from build123d import *

# Parameters (mm, degrees)
SKETCH1_R           = 0.75
SKETCH1_R_2         = 0.5
BOSS_EXTRUDE1_DEPTH = 2


with BuildPart() as part:
    # Sketch1 → Boss-Extrude1 (new body)
    with BuildSketch(Plane.XY):
        with BuildLine():
            Line((0, 16), (0, 14))
            Line((0, 14), (4, 14))
            Line((4, 14), (4, 12))
            Line((4, 12), (0, 12))
            Line((0, 12), (0, 6))
            Line((0, 6), (4, 6))
            Line((4, 6), (4, 4))
            Line((4, 4), (0, 4))
            Line((0, 4), (0, 2))
            ThreePointArc((0, 2), (0.585786438, 0.585786438), (2, 0))
            Line((2, 0), (14.2, 0))
            ThreePointArc((14.2, 0), (15.614213562, 0.585786438), (16.2, 2))
            Line((16.2, 2), (16.2, 4))
            Line((16.2, 4), (12.2, 4))
            Line((12.2, 4), (12.2, 6))
            Line((12.2, 6), (16.2, 6))
            Line((16.2, 6), (16.2, 12))
            Line((16.2, 12), (12.2, 12))
            Line((12.2, 12), (12.2, 14))
            Line((12.2, 14), (16.2, 14))
            Line((16.2, 14), (16.2, 16))
            ThreePointArc((16.2, 16), (14.735533906, 19.535533906), (11.2, 21))
            Line((11.2, 21), (5, 21))
            ThreePointArc((5, 21), (1.464466094, 19.535533906), (0, 16))
        make_face()
        with Locations((10.2, 8.5)):
            Circle(SKETCH1_R, mode=Mode.SUBTRACT)
        with Locations((6, 8.5)):
            Circle(SKETCH1_R, mode=Mode.SUBTRACT)
        with Locations((3, 18)):
            Circle(SKETCH1_R_2, mode=Mode.SUBTRACT)
        with Locations((13.2, 18)):
            Circle(SKETCH1_R_2, mode=Mode.SUBTRACT)
        with Locations((13.45, 2)):
            Circle(SKETCH1_R, mode=Mode.SUBTRACT)
        with Locations((2.75, 2)):
            Circle(SKETCH1_R, mode=Mode.SUBTRACT)
    extrude(amount=BOSS_EXTRUDE1_DEPTH)


solid = part.part
Can you work these out from the model? Positions are in its coordinate system, mm. A direction names the side the tool comes from. Coordinates: 2 decimals unless noted, no trailing zeros. Write each loop counter-clockwise with the first axis right and the second up, starting at its lowest first coordinate (ties: lowest second). Pieces come first, ordered by that corner, then holes. Notation, with made-up numbers: (14.25, 83.5) -> (49.25, 83.5) arc R20 cw to (49.25, 111.5) -> close; hole circle Ø4 at (79.5, -8.75). An arc over 180 degrees is marked (long way). Write item = value, one per line.
(1) On a 3-axis mill with a long thin cutter (end or side, diameter ignored), from which of +Z, -Z, +X, -X, +Y, -Y can I reach the whole of each face in a straight line? I mean faces 1 (the face through (8, 11, 2)), 2 (the face through (12.2, 13, 1)), 3 (the face through (2, 6, 1)). Say none if no direction works.
Verdict:
face_1 = +Z, +X, -X, +Y, -Y
face_2 = +Z, -Z, +X
face_3 = +Z, -Z, -X
(2) For pin 1 (0.6 mm diameter, centred on y = 12.5, z = 0.5, fed in from -X); pin 2 (1 mm diameter, centred on x = 2.5, z = 1, fed in from +Y); pin 3 (1 mm diameter, centred on x = 15, z = 0.5, fed in from +Y), each with a flat end and sliding along its axis, tell me the tip position at first contact or that it passes through.
Verdict:
pin_1 = 4
pin_2 = 20.58
pin_3 = 19.76
(3) Imagine slicing it at D-D (x = 2.75). Please give me the cut outline in (y, z), and give its area (3 significant figures).
Verdict:
outline = (0, 0) -> (1.25, 0) -> (1.25, 2) -> (0, 2) -> close; (2.75, 0) -> (4, 0) -> (4, 2) -> (2.75, 2) -> close; (6, 0) -> (12, 0) -> (12, 2) -> (6, 2) -> close; (14, 0) -> (17.57, 0) -> (17.57, 2) -> (14, 2) -> close; (18.43, 0) -> (20.47, 0) -> (20.47, 2) -> (18.43, 2) -> close
area = 28.2 mm^2
(4) Imagine slicing it at C-C (x = 6). Please give me the cut outline in (y, z), and give its area (3 significant figures).
Verdict:
outline = (0, 0) -> (7.75, 0) -> (7.75, 2) -> (0, 2) -> close; (9.25, 0) -> (21, 0) -> (21, 2) -> (9.25, 2) -> close
area = 39.0 mm^2
(5) If I drill on probe 1 along Y at (x, z) = (10.2, 0.8); probe 2 along Y at (x, z) = (14.25, 0.8); probe 3 along X at (y, z) = (13.75, 0.3), over which ranges is the centre line in solid material (lowest first)?
Verdict:
probe_1 = 0 to 7.75, 9.25 to 21
probe_2 = 0 to 4, 6 to 12, 14 to 19.96
probe_3 = 4 to 12.2
(6) Imagine slicing it at B-B (y = 8.5). Please give me the cut outline in (x, z), and give its area (3 significant figures).
Verdict:
outline = (0, 0) -> (5.25, 0) -> (5.25, 2) -> (0, 2) -> close; (6.75, 0) -> (9.45, 0) -> (9.45, 2) -> (6.75, 2) -> close; (10.95, 0) -> (16.2, 0) -> (16.2, 2) -> (10.95, 2) -> close
area = 26.4 mm^2
(7) Imagine slicing it at A-A (z = 1.45). State how many separate pieces and enclosed holes the cut face has, and give its area (3 significant figures).
Verdict:
separate_pieces = 1
enclosed_holes = 6
area = 287 mm^2
